from build123d import *

# Parameters (mm, degrees)
F1_DEPTH = 63.5
F0_W     = 25.4
F0_H     = 19.05
F2_DEPTH = 25.4
F3_DEPTH = 7.9375


with BuildPart() as f1:
    # F0 (on Front) → F1 (new body, symmetric)
    with BuildSketch(Plane.XZ):
        Polygon((41.275, -9.525), (41.275, 9.525), (22.225, 9.525), (-41.275, 9.525), (-41.275, -9.525), align=None)
    extrude(amount=F1_DEPTH, both=True)

    # F0 (on Front) → F2 (join, symmetric)
    with BuildSketch(Plane.XZ):
        with BuildLine():
            Line((22.225, 9.525), (41.275, 9.525))
            Line((41.275, 9.525), (41.275, 26.9875))
            ThreePointArc((41.275, 26.9875), (45.9246798487, 38.2128201513), (57.15, 42.8625))
            Line((57.15, 42.8625), (60.325, 42.8625))
            Line((60.325, 42.8625), (60.325, 61.9125))
            Line((60.325, 61.9125), (57.15, 61.9125))
            add(Edge.make_bspline(
                [(54.1562335502, 61.783950788), (55.1478189239, 61.8321045059), (56.1457632688, 61.8749746399), (57.15, 61.9125)],
                knots=[109.6652027071, 109.6652027071, 109.6652027071, 109.6652027071, 111.4985685166, 111.4985685166, 111.4985685166, 111.4985685166], degree=3))
            ThreePointArc((54.1562335502, 61.783950788), (31.4175990407, 50.6010377669), (22.225, 26.9875))
            Line((22.225, 26.9875), (22.225, 9.525))
        make_face()
        with Locations((73.025, 52.3875)):
            Rectangle(F0_W, F0_H)
    extrude(amount=F2_DEPTH, both=True)

    # F0 (on Front) → F3 (join, symmetric)
    with BuildSketch(Plane.XZ):
        with BuildLine():
            Line((-41.275, 9.525), (22.225, 9.525))
            Line((22.225, 9.525), (22.225, 26.9875))
            ThreePointArc((22.225, 26.9875), (31.4175990407, 50.6010377669), (54.1562335502, 61.783950788))
            add(Edge.make_bspline(
                [(-41.275, 9.525), (-41.7173976774, 37.118570419), (-5.1567581261, 58.9035724155), (54.1562335502, 61.783950788)],
                knots=[0, 0, 0, 0, 109.6652027071, 109.6652027071, 109.6652027071, 109.6652027071], degree=3))
        make_face()
    extrude(amount=F3_DEPTH, both=True)

    # F0 (on Front) → F4 (revolve)
    with BuildSketch(Plane.XZ):
        Polygon((85.725, 61.9125), (85.725, 42.8625), (85.725, 38.1), (111.125, 38.1), (111.125, 66.675), (85.725, 66.675), align=None)
    revolve(axis=Axis((85.725, 0, 52.3875), (0, 0, 1)))


solid = f1.part
Check sheet for the modelled part. Datum: model origin and axes. Units: mm. A direction names the side the tool comes from. Give positions to 0.01 mm unless a question says otherwise; leave off trailing zeros. Order: outer loops, then holes, each group sorted by start corner. A loop starts at its lowest first (then second) coordinate and runs counter-clockwise, first axis right, second up. Notation, with made-up numbers: M 56.25,-29.5 L 79.25,-29.5 A35 cw 79.25,9.5 Z; hole C 3.25,9 d4. An arc over 180 degrees is marked long. Answer as CSV lines item,"result". Start each with the question number.
Item 1: Thickness scan on line 1 (Z direction, x = 99.5, y = -16) (3 decimals); line 2 (Y direction, x = -24, z = 13); line 3 (X direction, y = 44, z = -5.5) (3 decimals). Record the ranges inside material, lowest first. Write a range as [from, to].
Item 2: Gauge pin test, flat ends, axial feed: P1, Ø3, axis at x = 82.5, y = 24.5, coming from the -Z side; P2, Ø2, axis at y = 8.5, z = 1.5, coming from the +X side (3 decimals); P3, Ø8, axis at y = 18.5, z = 36, coming from the -X side; P4, Ø10, axis at x = 42.5, z = 2.5, coming from the -Y side. Record the tip position at first contact, or that the pin passes through.
Item 3: Tool access check on faces 4 (the face through (-5, -7.938, 30)), 5 (the face through (1, 35, 9.525)), 6 (the face through (45.802, -0.356, 38.089)), 7 (the face through (60, -2, 61.912)), 8 (the face through (41.275, -1, 4)). Record the directions out of +Z, -Z, +X, -X, +Y, -Y that give a thin tool (end or side, any length) a straight path to the whole face; none if there is none.
Item 4: Cross-section at B-B on z = 3. Enter the section's corners in (x, y) (3 decimals).
Item 5: Cross-section at C-C on y = -30. Enter the section's corners in (x, z) (3 decimals).
Item 6: Cross-section at A-A on x = 65. Enter the section's corners in (y, z) (1 decimal).
Item 7: Mould release check, pull along X, two halves, no side actions. Record for faces 1 (the face through (46, 25.4, 42)), 2 (the face through (60, 2, 42.862)), 3 (the face through (22.225, -17, 18)): +X half, -X half, draft (parallel to the pull), parting line (faces both ways), or undercut.
Established:
1,line 1,"z = [38.1, 66.675]"
1,line 2,"y = [-7.94, 7.94]"
1,line 3,"x = [-41.275, 41.275]"
2,P1,"stops at z = 38.1"
2,P2,"stops at x = 41.275"
2,P3,"stops at x = 22.59"
2,P4,"stops at y = -63.5"
3,face 4,"+Z, -X, -Y"
3,face 5,"+Z, -X, +Y"
3,face 6,"-Z, +Y, -Y"
3,face 7,"+Z, -X"
3,face 8,"-Z, +X, +Y, -Y"
4,outline,"M -41.275,-63.5 L 41.275,-63.5 L 41.275,63.5 L -41.275,63.5 Z"
5,outline,"M -41.275,-9.525 L 41.275,-9.525 L 41.275,9.525 L -41.275,9.525 Z"
6,outline,"M -25.4,42.9 L -14.7,42.9 L -14.7,38.1 L 14.7,38.1 L 14.7,42.9 L 25.4,42.9 L 25.4,61.9 L 14.7,61.9 L 14.7,66.7 L -14.7,66.7 L -14.7,61.9 L -25.4,61.9 Z"
7,face 1,"draft"
7,face 2,"undercut"
7,face 3,"-X half"
